The model under review builds one solid part; all positions refer to its coordinate system, in mm. Coordinates: 2 decimals unless noted, no trailing zeros. Write each loop counter-clockwise with the first axis right and the second up, starting at its lowest first coordinate (ties: lowest second). Pieces come first, ordered by that corner, then holes. Notation, with made-up numbers: (34.5, 81.5) - (48.5, 81.5) arc R22 cw to (48.5, 98.5) - close; hole circle Ø2 at (16.25, 12.5). An arc over 180 degrees is marked (long way). Put each result on its own line as item: value. Start each with the question number.
Item 1: For pin 1 (1.3 mm diameter, centred on x = -1, y = -12, fed in from -Z); pin 2 (6 mm diameter, centred on x = 5.5, y = -3, fed in from -Z), all flat-tipped, find the tip position at first contact; note any pin that passes through.
Item 2: Consider section C-C on z = 134. Give the boundary of the cut face in (x, y).
Item 3: Consider section B-B on x = -1.5. Give the boundary of the cut face in (y, z).
Item 4: Consider section A-A on z = 0. Give the boundary of the cut face in (x, y).
Item 5: To check wall thickness, follow L1, parallel to Y at x = -1.75, z = 177; L2, parallel to Y at x = 11.7, z = 0. State the ranges of each line that lie inside material, in increasing order. Write a range as [from, to].
Autodesk Inventor part; units mm, degrees
ref_plane "YZ Plane" through (0, 0, 0) normal (1, 0, 0) x (0, 1, 0)
ref_plane "XZ Plane" through (0, 0, 0) normal (0, 1, 0) x (-1, 0, 0)
ref_plane "XY Plane" through (0, 0, 0) normal (0, 0, 1) x (1, 0, 0)
sketch "Sketch1" plane through (0, 0, 0) normal (0, 0, 1) x (1, 0, 0)
  line L0 (-12.7, -12.7) -> (12.7, -12.7)
  line L1 (12.7, -12.7) -> (12.7, 12.7)
  line L2 (12.7, 12.7) -> (-12.7, 12.7)
  line L3 (-12.7, 12.7) -> (-12.7, -12.7)
  line L4 (-12.7, -12.7) -> (12.7, 12.7) construction
  line L5 (12.7, -12.7) -> (-12.7, 12.7) construction
  line L6 (-11.1125, -11.1125) -> (11.1125, -11.1125)
  line L7 (11.1125, -11.1125) -> (11.1125, 11.1125)
  line L8 (11.1125, 11.1125) -> (-11.1125, 11.1125)
  line L9 (-11.1125, 11.1125) -> (-11.1125, -11.1125)
  line L10 (-11.1125, -11.1125) -> (11.1125, 11.1125) construction
  line L11 (11.1125, -11.1125) -> (-11.1125, 11.1125) construction
  point P0 (0, 0)
  dimension "d0" = 25.4
  dimension "d1" = 25.4
  dimension "d2" = 1.5875
extrude "Extrusion1" add sketch "Sketch1" along normal mid plane 558.8
sketch "Sketch2" plane through (-12.7, -12.7, 279.4) normal (-1, 0, 0) x (0, 0, 1)
  circle A0 centre (-279.4, 12.7) radius 7.9375
  line L0 (-558.8, 12.7) -> (0, 12.7) construction
  line L1 (0, 1.5875) -> (0, 23.8125) construction
  circle A1 centre (-546.1, 9.8186) radius 3.175
  line L2 (-546.1, 0) -> (-558.8, 0)
  arc A2 (-558.8, 12.7) -> (-546.1, 0) centre (-546.1, 12.7) ccw
  line L3 (-558.8, 12.7) -> (-558.8, 0)
  line L4 (-558.8, 25.4) -> (0, 25.4) construction
  line L5 (-279.4, 25.4) -> (-279.4, 0) construction
  arc A3 (-12.7, 0) -> (0, 12.7) centre (-12.7, 12.7) ccw
  arc A4 (0, 12.7) -> (-12.7, 25.4) centre (-12.7, 12.7) ccw
  line L6 (-12.7, 25.4) -> (0, 25.4)
  line L7 (0, 25.4) -> (0, 12.7)
  line L8 (0, 12.7) -> (0, 0)
  line L9 (0, 0) -> (-12.7, 0)
  line L10 (-558.8, 0) -> (-558.8, 25.4) construction
  line L11 (0, 0) -> (-558.8, 0) construction
  circle A5 centre (-546.1, 9.8186) radius 12.7 construction
  circle A6 centre (-12.7, 15.875) radius 4.7625
  circle A7 centre (-431.8, 12.7) radius 3.175
  dimension "d5" = 15.875
  dimension "d6" = 6.35
  dimension "d13" = 12.7
  dimension "d14" = 9.8186
  dimension "d15" = 25.4
  dimension "d19" = 9.525
  dimension "d20" = 12.7
  dimension "d21" = 9.525
  dimension "d22" = 6.35
  dimension "d23" = 127
extrude "Extrusion2" cut sketch "Sketch2" against normal through all
sketch "Sketch4" plane through (0, 0, 0) normal (0, 1, 0) x (-1, 0, 0)
  line L0 (-12.7, -266.7) -> (12.7, -266.7) construction
  line L1 (11.1125, -290.9216) -> (-11.1125, -290.9216)
  line L2 (-11.1125, -290.9216) -> (-11.1125, -254)
  line L3 (-11.1125, -254) -> (11.1125, -254)
  line L4 (11.1125, -254) -> (11.1125, -290.9216)
  line L5 (-11.1125, 272.8484) -> (11.1125, 272.8484) construction
  line L6 (11.1125, -279.4) -> (11.1125, 272.8484) construction
  line L7 (-11.1125, -279.4) -> (11.1125, -279.4) construction
  line L8 (-11.1125, -279.4) -> (-11.1125, 272.8484) construction
  point P0 (0, 0)
  dimension "d16" = 12.7
extrude "Extrusion4" cut sketch "Sketch4" against normal through all
properties part number "Front lift arm" material "Aluminum 6061"
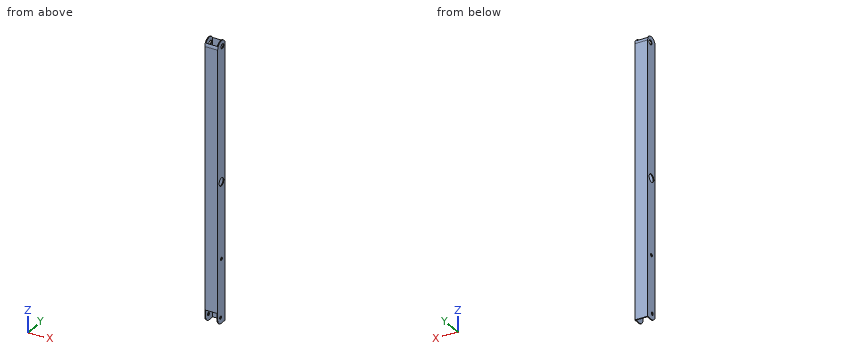
Report:
1. pin 1: z = -254
1. pin 2: through
2. outline: (-12.7, -12.7) - (12.7, -12.7) - (12.7, 12.7) - (-12.7, 12.7) - close; hole (-11.11, -11.11) - (11.11, -11.11) - (11.11, 11.11) - (-11.11, 11.11) - close
3. outline: (-12.7, -254) - (-11.11, -254) - (-11.11, 272.85) arc R12.7 ccw to (-12.7, 266.7) - close; (11.11, -279.4) - (12.7, -279.4) - (12.7, 266.7) arc R12.7 ccw to (11.11, 272.85) - close
4. outline: (-12.7, -12.7) - (12.7, -12.7) - (12.7, -7.94) - (11.11, -7.94) - (11.11, -11.11) - (-11.11, -11.11) - (-11.11, -7.94) - (-12.7, -7.94) - close; (-12.7, 7.94) - (-11.11, 7.94) - (-11.11, 11.11) - (11.11, 11.11) - (11.11, 7.94) - (12.7, 7.94) - (12.7, 12.7) - (-12.7, 12.7) - close
5. L1: [-12.7, -11.11], [11.11, 12.7]
5. L2: [-12.7, -7.94], [7.94, 12.7]
